Read the model definition and answer for the solid it produces. Units are mm, in the model's axes. Face numbers are marked on the shaded views. Coordinates: 2 decimals unless noted, no trailing zeros. Write each loop counter-clockwise with the first axis right and the second up, starting at its lowest first coordinate (ties: lowest second). Pieces come first, ordered by that corner, then holes. Notation, with made-up numbers: (87.25, 59.5) -> (133.25, 59.5) arc R21 ccw to (133.25, 86.5) -> close; hole circle Ø3 at (8.5, 77). An arc over 180 degrees is marked (long way). Write item = value, one per line. Start each with the question number.
1) Section A-A (y = 16.25) is taken. Determine the outline of the cut face in (x, z).
2) Section C-C (y = 8) is taken. Determine the outline of the cut face in (x, z).
3) Section B-B (x = -50) is taken. Determine the outline of the cut face in (y, z).
4) Find the intervals of material crossed by line 1 along Z through (x, y) = (-50, 17.5); line 2 along Y through (x, z) = (7.5, 10.75); line 3 along Y through (x, z) = (-37.5, 14.5), in increasing order. Write a range as from..to.
5) Section D-D (z = 17) is taken. Determine the outline of the cut face in (x, y).
6) For a pull along X with two mould halves and no side action, classify the marked faces 1, 2 and 3 as released by +X, released by -X, zero draft, split by the parting line, or undercut.
7) Flat-ended cylindrical pins translate along their axes: pin 1 Ø10 at (x, z) = (23, 2) entering from -Y; pin 2 Ø8 at (x, z) = (54.5, 8.5) entering from -Y; pin 3 Ø4 at (x, z) = (-33.5, 15) entering from -Y; pin 4 Ø5.5 at (x, z) = (-50, 17) entering from +Y. Find the tip coordinate at first contact, or state that the pin passes through.
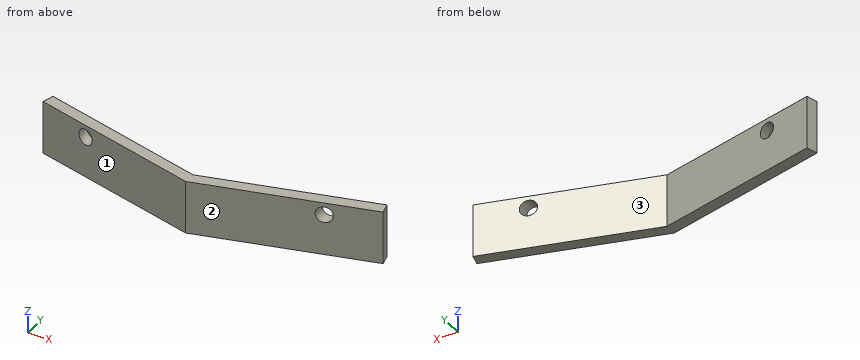
from build123d import *

# Parameters (mm, degrees)
F1_DEPTH = 22
F3_D     = 6.6


with BuildPart() as f1:
    # F0 (on Top) → F1 (new body)
    with BuildSketch(Plane.XY):
        Polygon((-70, 23.9328243722), (-71.2940952255, 19.1031952408), (0, 0), (71.2940952255, 19.1031952408), (70, 23.9328243722), (0, 5.1763809021), align=None)
    extrude(amount=F1_DEPTH)

    # F3 (through all)
    with Locations(Plane.XZ):
        with Locations((-50, 17), (50, 17)):
            Hole(F3_D / 2)


solid = f1.part
Answer key:
q1.outline = (-60.65, 0) -> (-41.33, 0) -> (-41.33, 22) -> (-60.65, 22) -> close; (41.33, 0) -> (60.65, 0) -> (60.65, 22) -> (41.33, 22) -> close; hole circle Ø6.6 at (-50, 17); hole circle Ø6.6 at (50, 17)
q2.outline = (-29.86, 0) -> (-10.54, 0) -> (-10.54, 22) -> (-29.86, 22) -> close; (10.54, 0) -> (29.86, 0) -> (29.86, 22) -> (10.54, 22) -> close
q3.outline = (13.4, 0) -> (18.57, 0) -> (18.57, 13.7) -> (13.4, 13.7) -> close; (13.4, 20.3) -> (18.57, 20.3) -> (18.57, 22) -> (13.4, 22) -> close
q4.line_1 = 0..13.7, 20.3..22
q4.line_2 = 2.01..7.19
q4.line_3 = 10.05..15.22
q5.outline = (-71.29, 19.1) -> (-53.3, 14.28) -> (-53.3, 19.46) -> (-70, 23.93) -> close; (-46.7, 12.51) -> (0, 0) -> (46.7, 12.51) -> (46.7, 17.69) -> (0, 5.18) -> (-46.7, 17.69) -> close; (53.3, 14.28) -> (71.29, 19.1) -> (70, 23.93) -> (53.3, 19.46) -> close
q6.face_1 = released by -X
q6.face_2 = released by +X
q6.face_3 = undercut
q7.pin_1 = 4.82
q7.pin_2 = 13.53
q7.pin_3 = 8.44
q7.pin_4 = through
